```python
from build123d import *

# Parameters (mm, degrees)
F1_DEPTH                 = 2
F0_R                     = 2.5
F0_W                     = 1.9671103259
F0_H                     = 32.8726123017
F2_DEPTH                 = 23
F3_DEPTH                 = 21
F3_FACE_W                = 2
F3_FACE_H                = 47.3760884154
FLPUHT3DEIL0ECL_2_FACE_W = 9.4088794868
FLPUHT3DEIL0ECL_2_FACE_H = 2
F5_DEPTH                 = 2
F5_FACE_W                = 9.4088794868
F5_FACE_H                = 2
F7_R                     = 1


with BuildPart() as f1:
    # F0 (on Front) → F1 (new body)
    with BuildSketch(Plane.XZ):
        Polygon((-27.4859799968, -94.5354314736), (-36.8948594836, -94.5354314736), (-29.0944709842, -132.4704811186), (-24.7819819802, -132.2534833467), align=None)
    extrude(amount=-F1_DEPTH)



with BuildPart() as f2:
    # F0 (on Front) → F2 (new body, symmetric)
    with BuildSketch(Plane.XZ):
        with BuildLine():
            Line((-57.4354853918, 38.2308801777), (-57.4354853918, 5.358267876))
            Line((-57.4354853918, 5.358267876), (-31.1536770314, -34.0594984591))
            add(Edge.make_bspline(
                [(-21.304015945, 20.5783754124), (-34.3524827141, 3.69984575), (-31.5767975227, -1.8766191306), (-31.1536770314, -34.0594984591)],
                knots=[0, 0, 0, 0, 56.0586211891, 56.0586211891, 56.0586211891, 56.0586211891], degree=3))
            Line((-21.304015945, 20.5783754124), (-19.717078656, 30.4542761296))
            Line((-19.717078656, 30.4542761296), (-25.1840222627, 40.1536934078))
            add(Edge.make_bspline(
                [(-41.9375598431, 64.1377046704), (-34.8834395409, 55.6727573276), (-36.6469696164, 50.3821708262), (-25.1840222627, 40.1536934078)],
                knots=[0, 0, 0, 0, 29.2560048145, 29.2560048145, 29.2560048145, 29.2560048145], degree=3))
            add(Edge.make_bspline(
                [(-41.9375598431, 64.1377046704), (-51.2842722237, 47.7368719876), (-55.3985677235, 50.4242394975), (-57.4354853918, 38.2308801777)],
                knots=[0, 0, 0, 0, 30.1885616022, 30.1885616022, 30.1885616022, 30.1885616022], degree=3))
        make_face()
        with Locations((-36.313764751, 30.7701863348)):
            Circle(F0_R, mode=Mode.SUBTRACT)
        with Locations((-58.4190405548, 21.7945740269)):
            Rectangle(F0_W, F0_H)
    extrude(amount=F2_DEPTH, both=True)

    # F0 (on Front) → F3 (cut, symmetric)
    with BuildSketch(Plane.XZ):
        with BuildLine():
            Line((-57.4354853918, 38.2308801777), (-57.4354853918, 5.358267876))
            Line((-57.4354853918, 5.358267876), (-31.1536770314, -34.0594984591))
            add(Edge.make_bspline(
                [(-21.304015945, 20.5783754124), (-34.3524827141, 3.69984575), (-31.5767975227, -1.8766191306), (-31.1536770314, -34.0594984591)],
                knots=[0, 0, 0, 0, 56.0586211891, 56.0586211891, 56.0586211891, 56.0586211891], degree=3))
            Line((-21.304015945, 20.5783754124), (-19.717078656, 30.4542761296))
            Line((-19.717078656, 30.4542761296), (-25.1840222627, 40.1536934078))
            add(Edge.make_bspline(
                [(-41.9375598431, 64.1377046704), (-34.8834395409, 55.6727573276), (-36.6469696164, 50.3821708262), (-25.1840222627, 40.1536934078)],
                knots=[0, 0, 0, 0, 29.2560048145, 29.2560048145, 29.2560048145, 29.2560048145], degree=3))
            add(Edge.make_bspline(
                [(-41.9375598431, 64.1377046704), (-51.2842722237, 47.7368719876), (-55.3985677235, 50.4242394975), (-57.4354853918, 38.2308801777)],
                knots=[0, 0, 0, 0, 30.1885616022, 30.1885616022, 30.1885616022, 30.1885616022], degree=3))
        make_face()
        with Locations((-36.313764751, 30.7701863348)):
            Circle(F0_R, mode=Mode.SUBTRACT)
    extrude(amount=F3_DEPTH, both=True, mode=Mode.SUBTRACT)


with BuildPart() as f1_1:
    add(f1.part)

    add(f2.part)  # F4 merges F2
    # F3_face (on face) → F4 section 0
    with BuildSketch(Plane(origin=(-44.2945812116, 22, -14.3506152915), x_dir=(0, -1, 0), z_dir=(-0.8320181689, 0, -0.5547483813))):
        Rectangle(F3_FACE_W, F3_FACE_H)
    # FlpuHt3dEil0ecl_2_face (on face) → F4 section 1
    with BuildSketch(Plane(origin=(-32.1904197402, 1, -94.5354314736), x_dir=(1, 0, 0), z_dir=(0, 0, 1))):
        Rectangle(FLPUHT3DEIL0ECL_2_FACE_W, FLPUHT3DEIL0ECL_2_FACE_H)
    loft()

    # F0 (on Front) → F5 (join)
    with BuildSketch(Plane.XZ):
        Polygon((-27.4859799968, -94.5354314736), (-36.8948594836, -94.5354314736), (-29.0944709842, -132.4704811186), (-24.7819819802, -132.2534833467), align=None)
    extrude(amount=F5_DEPTH)

    # F3_face (on face) → F6 section 0
    with BuildSketch(Plane(origin=(-44.2945812116, 22, -14.3506152915), x_dir=(0, -1, 0), z_dir=(-0.8320181689, 0, -0.5547483813))):
        with Locations((44, 0)):
            Rectangle(F3_FACE_W, F3_FACE_H)
    # F5_face (on face) → F6 section 1
    with BuildSketch(Plane(origin=(-32.1904197402, -1, -94.5354314736), x_dir=(1, 0, 0), z_dir=(0, 0, 1))):
        Rectangle(F5_FACE_W, F5_FACE_H)
    loft()

    # F7
    f7_edges = [f1_1.edges().sort_by_distance(p)[0] for p in [
        (-59.402596, -23, 21.794574),
        (-59.402596, 23, 21.794574),
    ]]
    fillet(f7_edges, radius=F7_R)


solid = f1_1.part
```
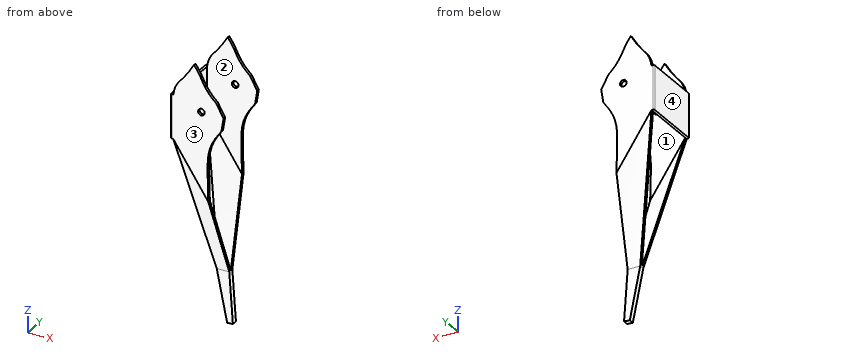
Verification items for the finished model (mm, model axes). Face numbers are marked on the shaded views. Coordinates: 2 decimals unless noted, no trailing zeros. Order: outer loops, then holes, each group sorted by start corner. A loop starts at its lowest first (then second) coordinate and runs counter-clockwise, first axis right, second up. Notation, with made-up numbers: (65, -16) -> (102, -16) arc R17 cw to (102, 4) -> close; hole circle Ø11 at (85.5, 62.25). An arc over 180 degrees is marked (long way). Put each result on its own line as item: value. Start each with the question number.
1) Material ranges on L1, parallel to Y at x = -31, z = 38.5; L2, parallel to Y at x = -32.5, z = -52; L3, parallel to X at y = 2.5, z = 33.5, recorded low to high.
2) Cross-section at A-A (z = 22.5). Enter the section's corners in (x, y).
3) Go/stop test with flat-tipped pins: pin 1 (1 mm diameter, centred on x = -58, y = 0, fed in from +Z); pin 2 (0.6 mm diameter, centred on x = -59, y = -6.5, fed in from -Z); pin 3 (9.5 mm diameter, centred on x = -29, z = -107, fed in from -Y); pin 4 (8 mm diameter, centred on y = -9, z = 43.5, fed in from +X). Record where each tip stops, or that it passes through.
4) Release check for a two-part mould opening along Y. For the marked faces 1, 2, 3 and 4 record: pulls with the +Y half, pulls with the -Y half, needs draft (parallel to the pull), parting line crosses it, or undercut.
Geometry check:
1. L1: y = -23 to -21, 21 to 23
1. L2: y = -15.62 to -13.62, 13.62 to 15.62
1. L3: x = -59.4 to -57.44
2. outline: (-59.4, -22) arc R1 ccw to (-58.4, -23) -> (-21, -23) -> (-21, -21) -> (-57.44, -21) -> (-57.44, 21) -> (-21, 21) -> (-21, 23) -> (-58.4, 23) arc R1 ccw to (-59.4, 22) -> close
3. pin 1: stops at z = 38.23
3. pin 2: stops at z = 5.36
3. pin 3: stops at y = -2
3. pin 4: passes through
4. face 1: undercut
4. face 2: undercut
4. face 3: pulls with the -Y half
4. face 4: needs draft
